from build123d import *

# Parameters (mm, degrees)
BOSS_EXTRUDE1_DEPTH = 0.8
FILLET1_R           = 0.1


with BuildPart() as part:
    # Sketch1 → Boss-Extrude1 (new body)
    with BuildSketch(Plane(origin=(0, 0, 0), x_dir=(1, 0, 0), z_dir=(0, 1, 0))):
        with BuildLine():
            ThreePointArc((8.734573904, -7.933928328), (2.023691137, 11.625174157), (-10.901778484, -4.515664502))
            ThreePointArc((-10.901778484, -4.515664502), (-9.670610732, -4.932925102), (-8.73153967, -5.831827757))
            ThreePointArc((-8.73153967, -5.831827757), (-1.800742113, -10.344434631), (6.247243618, -8.439309639))
            ThreePointArc((6.247243618, -8.439309639), (7.434829013, -7.910611831), (8.734573904, -7.933928328))
        make_face()
        with BuildLine():
            Line((-1.5, 6.5), (1.5, 6.5))
            Line((1.5, 6.5), (1.5, 7.858116823))
            ThreePointArc((1.5, 7.858116823), (0, -8), (-1.5, 7.858116823))
            Line((-1.5, 7.858116823), (-1.5, 6.5))
        make_face(mode=Mode.SUBTRACT)
    extrude(amount=BOSS_EXTRUDE1_DEPTH)

    # Fillet1
    fillet1_edges = [part.edges().sort_by_distance(p)[0] for p in [
        (-1.5, 0.4, -7.858116823),
        (1.5, 0.4, -7.858116823),
    ]]
    fillet(fillet1_edges, radius=FILLET1_R)


solid = part.part
Can you work these out from the model? Positions are in its coordinate system, mm. Give positions to 0.01 mm unless a question says otherwise; leave off trailing zeros. Write each loop counter-clockwise with the first axis right and the second up, starting at its lowest first coordinate (ties: lowest second). Pieces come first, ordered by that corner, then holes. Notation, with made-up numbers: M -24.5,10 L 7.5,10 A20 ccw 7.5,25 Z; hole C 59.5,-30 d2. An arc over 180 degrees is marked long. Answer in a Markdown table with one row per item. Add a question column.
Item 1: Imagine slicing it at B-B, the plane y = 0.4. Write out the boundary of the cut face in (x, z), plus the area to 3 significant figures.
Item 2: For pin 1 Ø12 at (x, z) = (0, -1.5) entering from -Y, with a flat end and sliding along its axis, tell me the tip position at first contact or that it passes through.
Item 3: We'd pull the mould along X, two halves only. Please class faces 1 (the cylindrical face through (0.329, 0.394, 7.993)), 2 (the flat face through (0, 0, -8)), 3 (the cylindrical face through (-1.918, 0.394, 10.323)): released by +X, released by -X, zero draft, split by the parting line, or undercut.
Item 4: Please list where these lines run through material, in increasing order: L1, parallel to X at y = 0.65, z = 0; L2, parallel to Z at x = 0.25, y = 0.7; L3, parallel to Z at x = 2.5, y = 0.75.
Item 5: Imagine slicing it at C-C, the plane z = 0. Write out the boundary of the cut face in (x, y).
Item 6: Imagine slicing it at D-D, the plane x = -9.25. Write out the boundary of the cut face in (y, z), plus the area to 3 significant figures.
Item 7: Imagine slicing it at A-A, the plane x = 0. Write out the boundary of the cut face in (y, z), plus the area to 3 significant figures.
Evaluation:
| question | item | result |
|---|---|---|
| 1 | outline | M -10.9,4.52 A11.8 ccw long 8.73,7.93 A3 cw 6.25,8.44 A10.5 ccw -8.73,5.83 A3 cw Z; hole M -1.62,-7.83 A0.1 ccw -1.5,-7.74 L -1.5,-6.5 L 1.5,-6.5 L 1.5,-7.74 A0.1 ccw 1.62,-7.83 A8 ccw long Z |
| 1 | area | 213 mm² |
| 2 | pin 1 | stops at y = 0 |
| 3 | face 1 | undercut |
| 3 | face 2 | zero draft |
| 3 | face 3 | split by the parting line |
| 4 | L1 | x = -11.8 to -8, 8 to 11.8 |
| 4 | L2 | z = -11.8 to -6.5, 8 to 10.5 |
| 4 | L3 | z = -11.53 to -7.6, 7.6 to 10.2 |
| 5 | outline | M -11.8,0 L -8,0 L -8,0.8 L -11.8,0.8 Z; M 8,0 L 11.8,0 L 11.8,0.8 L 8,0.8 Z |
| 6 | outline | M 0,-7.33 L 0.8,-7.33 L 0.8,5.24 L 0,5.24 Z |
| 6 | area | 10.1 mm² |
| 7 | outline | M 0,-11.8 L 0.8,-11.8 L 0.8,-6.5 L 0,-6.5 Z; M 0,8 L 0.8,8 L 0.8,10.5 L 0,10.5 Z |
| 7 | area | 6.24 mm² |
